Verification items for this drawing (mm, ordinates from the low corner). Give positions to 0.01 mm unless a question says otherwise; leave off trailing zeros. Write each loop counter-clockwise with the first axis right and the second up, starting at its lowest first coordinate (ties: lowest second). Pieces come first, ordered by that corner, then holes. Notation, with made-up numbers: M 74,-11 L 128,-11 A22 cw 128,17 Z; hole C 23,39 d1. An arc over 180 degrees is marked long. Use one line per item in the form item = value. Start each with the question number.
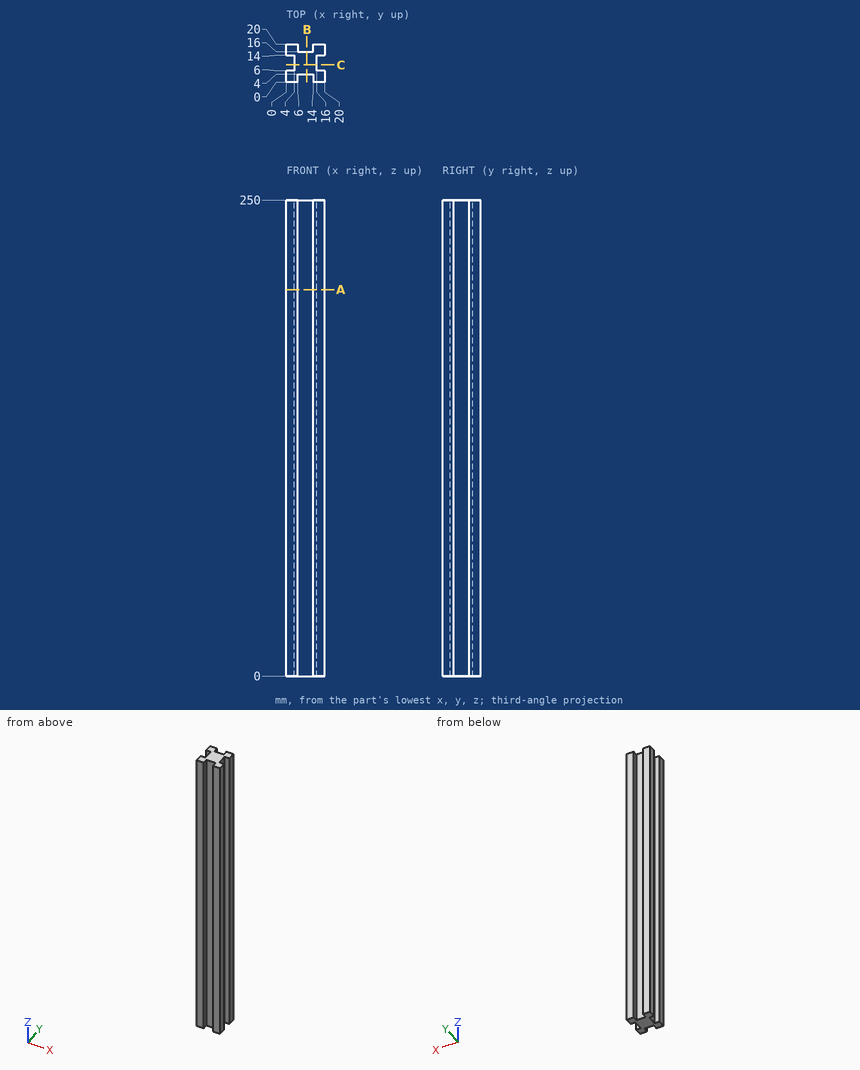
(1) Depth check by flat-ended pin: pin 1 (2.5 mm diameter, centred on x = 8.5, z = 179.5, fed in from +Y); pin 2 (4 mm diameter, centred on y = 9.5, z = 122.5, fed in from +X); pin 3 (1.5 mm diameter, centred on y = 11, z = 92, fed in from -X). Enter the tip coordinate at first touch or a pass-through.
(2) Sectioned sample at A-A, the plane z = 203. Record the boundary of the cut face in (x, y), plus the area to 3 significant figures.
(3) Sectioned sample at B-B, the plane x = 10.75. Record the boundary of the cut face in (y, z), plus the area to 3 significant figures.
(4) Thickness scan on probe 1 along X at (y, z) = (16.25, 117); probe 2 along X at (y, z) = (13, 192). Record the ranges inside material, lowest first. Write a range as [from, to].
Numbers:
q1.pin_1 = 16
q1.pin_2 = 16
q1.pin_3 = 4
q2.outline = M 0,0 L 6,0 L 6,4 L 14,4 L 14,0 L 20,0 L 20,6 L 16,6 L 16,14 L 20,14 L 20,20 L 14,20 L 14,16 L 6,16 L 6,20 L 0,20 L 0,14 L 4,14 L 4,6 L 0,6 Z
q2.area = 272 mm2
q3.outline = M 4,0 L 16,0 L 16,250 L 4,250 Z
q3.area = 3,000 mm2
q4.probe_1 = [0, 6], [14, 20]
q4.probe_2 = [4, 16]
